Model file for the job. Use its own axes, mm. Face numbers are marked on the shaded views. A direction names the side the tool comes from. Give positions to 0.01 mm unless a question says otherwise; leave off trailing zeros. Order: outer loops, then holes, each group sorted by start corner. A loop starts at its lowest first (then second) coordinate and runs counter-clockwise, first axis right, second up. Notation, with made-up numbers: M 85,-6 L 105,-6 A20 ccw 105,16 Z; hole C 10.25,24 d7. An arc over 180 degrees is marked long. Return JSON: item names as keys, results as strings. Group by question number.
1. Two-plate mould, pull along Z, no slides. Class the marked faces 1, 2, 3 and 4: released by +Z, released by -Z, zero draft, split by the parting line, or undercut.
2. Slice it at A-A on x = -2.25. List the corners of the cut face in (y, z).
3. Slice it at B-B on x = 11.25. List the corners of the cut face in (y, z), then the cut area to 3 significant figures.
4. Pin check, flat tips, straight feed: pin 1 (5 mm diameter, centred on x = 12.5, z = 3.5, fed in from +Y); pin 2 (1.4 mm diameter, centred on y = 0.5, z = -2, fed in from -X); pin 3 (1.2 mm diameter, centred on x = -3, y = 0.5, fed in from +Z); pin 4 (5 mm diameter, centred on x = 1.5, y = 2.5, fed in from -Z). Stop position of each tip, or through.
5. Wall check: probe 1 along Z at (x, y) = (0.3, 0); probe 2 along X at (y, z) = (-3.5, -1.5). Give the ranges that are in metal, low to high. Write a range as [from, to].
6. 3-axis set-ups, long thin cutter, end or side, ignore diameter. For the marked faces 5 and 6: which of +Z, -Z, +X, -X, +Y, -Y reach the whole face in a straight line?
from build123d import *

# Parameters (mm, degrees)
CUT_EXTRUDE1_DEPTH = 2.5


with BuildPart() as part:
    # Sketch1 → Revolve1 (revolve)
    with BuildSketch(Plane.XY):
        with BuildLine():
            Line((2.5, 0), (1, 1.5))
            Line((1, 1.5), (-0.5, 1.5))
            Line((-0.5, 1.5), (-1.5, 2.5))
            Line((-1.5, 2.5), (-3.613248654, 2.5))
            Line((-3.613248654, 2.5), (-4, 2.886751346))
            Line((-4, 2.886751346), (-4, 4.5))
            ThreePointArc((-4, 4.5), (-3.853553391, 4.853553391), (-3.5, 5))
            Line((-3.5, 5), (-0.5, 5))
            ThreePointArc((-0.5, 5), (-0.146446609, 4.853553391), (0, 4.5))
            Line((0, 4.5), (0, 3))
            Line((0, 3), (17.3865, 3))
            Line((17.3865, 3), (18, 2.3865))
            Line((18, 2.3865), (18, 0))
            Line((18, 0), (2.5, 0))
        make_face()
    revolve(axis=Axis((18, 0, 0), (-1, 0, 0)))

    # Sketch2 → Cut-Extrude1 (cut)
    with BuildSketch(Plane(origin=(-4, 0, 0), x_dir=(0, 0, -1), z_dir=(1, 0, 0))):
        Polygon((-2.5, -1.443375673), (0, -2.886751346), (2.5, -1.443375673), (2.5, 1.443375673), (0, 2.886751346), (-2.5, 1.443375673), align=None)
    extrude(amount=CUT_EXTRUDE1_DEPTH, mode=Mode.SUBTRACT)


solid = part.part
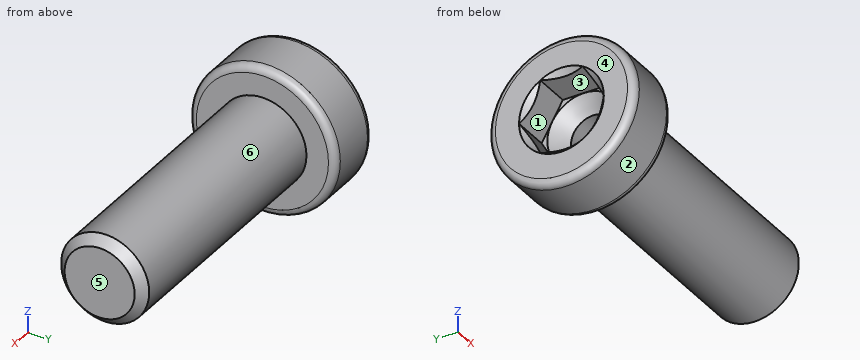
Result:
{
 "1": {"face 1": "undercut", "face 2": "split by the parting line", "face 3": "undercut", "face 4": "zero draft"},
 "2": {"outline": "C 0,0 d10; hole M -2.89,0 L -1.44,-2.5 L 1.44,-2.5 L 2.89,0 L 1.44,2.5 L -1.44,2.5 Z"},
 "3": {"outline": "C 0,0 d6", "area": "28.3 mm2"},
 "4": {"pin 1": "stops at y = 2.83", "pin 2": "stops at x = -3.87", "pin 3": "stops at z = 5", "pin 4": "stops at z = -4.91"},
 "5": {"probe 1": "z = [-3, -1.5], [1.5, 3]", "probe 2": "x = [-4, 0]"},
 "6": {"face 5": "+Z, -Z, +X, +Y, -Y", "face 6": "+X"}
}
